Work out the finished part from the listing and answer in its coordinate system (mm). A direction names the side the tool comes from. Give positions to 0.01 mm unless a question says otherwise; leave off trailing zeros. Write each loop counter-clockwise with the first axis right and the second up, starting at its lowest first coordinate (ties: lowest second). Pieces come first, ordered by that corner, then holes. Notation, with made-up numbers: (53, 57) -> (60, 57) arc R28 ccw to (60, 87) -> close; hole circle Ø9 at (13.5, -5.5). An arc over 180 degrees is marked (long way). Write item = value, one per line. Start each with the question number.
Autodesk Inventor part; units mm, degrees
ref_plane "YZ Plane" through (0, 0, 0) normal (1, 0, 0) x (0, 1, 0)
ref_plane "XZ Plane" through (0, 0, 0) normal (0, 1, 0) x (-1, 0, 0)
ref_plane "XY Plane" through (0, 0, 0) normal (0, 0, 1) x (1, 0, 0)
sketch "Sketch1" plane through (0, 0, 0) normal (0, 0, 1) x (1, 0, 0)
  line L0 (9, 0) -> (10, 0)
  line L1 (13, 0) -> (13, -10)
  line L2 (0, -13.9226) -> (0, -8.7389) construction
  line L3 (0.9, -13.9226) -> (0.9, -9.3264) construction
  line L4 (-0.7394, -10) -> (2.996, -10) construction
  line L5 (-0.7394, -9) -> (2.996, -9) construction
  line L6 (-0.7394, -5) -> (10, -5) construction
  line L7 (1.1988, -8.8687) -> (9.7012, -5.1313)
  line L8 (0.2988, -8.2812) -> (8.7012, -4.5878)
  arc A0 (0.2988, -8.2812) -> (0, -8.7389) centre (0.5, -8.7389) ccw
  arc A1 (1.1988, -8.8687) -> (0.9, -9.3264) centre (1.4, -9.3264) ccw
  line L9 (0.9, -9.3264) -> (0.9, -10)
  line L10 (0.9, -10) -> (0, -10)
  line L11 (10, 0) -> (10, -4.6736)
  line L12 (10, -13.9226) -> (10, -10) construction
  line L13 (10, -5) -> (10, 0) construction
  line L14 (9, 0) -> (9, -4.1301)
  line L15 (0, -8.7389) -> (0, -10)
  arc A2 (8.7012, -4.5878) -> (9, -4.1301) centre (8.5, -4.1301) ccw
  arc A3 (9.7012, -5.1313) -> (10, -4.6736) centre (9.5, -4.6736) ccw
  point P0 (0, 0)
  point P1 (0, -6.4341)
  point P2 (0.9, -9)
  dimension "d0" = 13
  dimension "d1" = 10
  dimension "d2" = 0.9
  dimension "d3" = 1
  dimension "d5" = 4
  dimension "d6" = 0.9
  dimension "d7" = 0.5
  dimension "d8" = 1
  dimension "d9" = 0.5
extrude "Extrusion1" add sketch "Sketch1" along normal blind 3.9
properties part number "Limit switch sheet" material "Silver"
(1) Find the intervals of material crossed by line 1 along X through (y, z) = (-2.5, 1.3); line 2 along X through (y, z) = (-9, 2.6); line 3 along Y through (x, z) = (1, 3.7), in increasing order.
(2) Each of these flat-tipped pins is pushed along its axis until it touches: pin 1 (0.5 mm diameter, centred on y = -10, z = 2, fed in from +X); pin 2 (1 mm diameter, centred on x = 2, z = 2.5, fed in from +Y). Where does it stop, or does it pass through?
(3) A cutting plane is placed at C-C, the plane x = 5.5. Write down the section's boundary in (y, z), then the cut area to 3 significant figures.
(4) For faces 1 (the flat face through (6, -6, 0)), 2 (the flat face through (9, -2, 2)), determine the directions among +Z, -Z, +X, -X, +Y, -Y from which every point of the face is accessible in a straight line to the end or side of a thin tool.
(5) A cutting plane is placed at A-A, the plane z = 2.4. Write down the section's boundary in (x, y).
(6) A cutting plane is placed at B-B, the plane y = -3.75. Write down the section's boundary in (x, z).
Results list:
q1.line_1 = 9 to 10
q1.line_2 = 0 to 1.02
q1.line_3 = -9.03 to -7.97
q2.pin_1 = 0.9
q2.pin_2 = -7.31
q3.outline = (-6.98, 0) -> (-5.99, 0) -> (-5.99, 3.9) -> (-6.98, 3.9) -> close
q3.area = 3.83 mm²
q4.face_1 = -Z, +X, -X, +Y, -Y
q4.face_2 = +Z, -Z, -X, +Y
q5.outline = (0, -10) -> (0.9, -10) -> (0.9, -9.33) arc R0.5 cw to (1.2, -8.87) -> (9.7, -5.13) arc R0.5 ccw to (10, -4.67) -> (10, 0) -> (9, 0) -> (9, -4.13) arc R0.5 cw to (8.7, -4.59) -> (0.3, -8.28) arc R0.5 ccw to (0, -8.74) -> close
q6.outline = (9, 0) -> (10, 0) -> (10, 3.9) -> (9, 3.9) -> close
